Source: CAD feature listing. Evaluate the final solid. Frame: model axes, mm. Round coordinates to 2 decimals unless told otherwise and drop trailing zeros. Order: outer loops, then holes, each group sorted by start corner. A loop starts at its lowest first (then second) coordinate and runs counter-clockwise, first axis right, second up. Notation, with made-up numbers: (-6, 23.25) -> (18, 23.25) arc R21 cw to (18, 56.25) -> close; hole circle Ø3 at (-23.5, 47.5). An arc over 180 degrees is marked (long way). Answer as CSV lines item,"result". Start each with the question number.
(1) Section query C-C (z = -38.5). Count the separate pieces of the cut face and the enclosed holes in it, plus the area to 3 significant figures.
(2) Line query: line 1 along Y through (x, z) = (0, -21.25); line 2 along X through (y, z) = (100, -43); line 3 along X through (y, z) = (20, -22). Output: solid intervals per line, ascending. Write a range as from..to.
(3) Section query B-B (x = 80). Output: boundary loops of the cut face in (y, z).
(4) Section query A-A (y = 59). Output: boundary loops of the cut face in (x, z).
(5) Contact query for flat-ended pins moving along their axis: P1, Ø7.5, axis at x = -80, y = 100, coming from the +Z side; P2, Ø15, axis at x = -80, y = 100, coming from the +Z side; P3, Ø16.5, axis at x = 160, y = 100, coming from the +Z side. Output: stop coordinate, or through.
```python
from build123d import *

# Parameters (mm, degrees)
F0_W     = 400
F0_H     = 120
F0_R     = 12.7
F0_R_2   = 6.35
F1_DEPTH = 60
F3_D     = 12
F3_DEPTH = 80
F3_TIP   = 3.6051637142
F4_D     = 25.4
F4_DEPTH = 30
F4_TIP   = 7.6309298617
F5_D     = 12.7


with BuildPart() as f1:
    # F0 (on Top) → F1 (new body)
    with BuildSketch(Plane.XY):
        with Locations((0, 60)):
            Rectangle(F0_W, F0_H)
        with Locations((-80, 20)):
            Circle(F0_R, mode=Mode.SUBTRACT)
        with Locations((0, 20)):
            Circle(F0_R, mode=Mode.SUBTRACT)
        with Locations((80, 20)):
            Circle(F0_R, mode=Mode.SUBTRACT)
        with Locations((160, 20)):
            Circle(F0_R, mode=Mode.SUBTRACT)
        with Locations((-160, 100)):
            Circle(F0_R, mode=Mode.SUBTRACT)
        with Locations((-80, 100)):
            Circle(F0_R, mode=Mode.SUBTRACT)
        with Locations((0, 100)):
            Circle(F0_R, mode=Mode.SUBTRACT)
        with Locations((80, 100)):
            Circle(F0_R, mode=Mode.SUBTRACT)
        with Locations((160, 100)):
            Circle(F0_R, mode=Mode.SUBTRACT)
        with Locations((-160, 100)):
            Circle(F0_R)
        with Locations((-160, 100)):
            Circle(F0_R_2, mode=Mode.SUBTRACT)
        with Locations((-80, 100)):
            Circle(F0_R)
        with Locations((-80, 100)):
            Circle(F0_R_2, mode=Mode.SUBTRACT)
        with Locations((0, 100)):
            Circle(F0_R)
        with Locations((0, 100)):
            Circle(F0_R_2, mode=Mode.SUBTRACT)
        with Locations((80, 100)):
            Circle(F0_R)
        with Locations((80, 100)):
            Circle(F0_R_2, mode=Mode.SUBTRACT)
        with Locations((160, 100)):
            Circle(F0_R)
        with Locations((160, 100)):
            Circle(F0_R_2, mode=Mode.SUBTRACT)
        with Locations((80, 20)):
            Circle(F0_R)
        with Locations((80, 20)):
            Circle(F0_R_2, mode=Mode.SUBTRACT)
        with Locations((160, 20)):
            Circle(F0_R)
        with Locations((160, 20)):
            Circle(F0_R_2, mode=Mode.SUBTRACT)
        with Locations((0, 20)):
            Circle(F0_R)
        with Locations((0, 20)):
            Circle(F0_R_2, mode=Mode.SUBTRACT)
        with Locations((-80, 20)):
            Circle(F0_R)
        with Locations((-80, 20)):
            Circle(F0_R_2, mode=Mode.SUBTRACT)
        with Locations((-160, 100)):
            Circle(F0_R_2)
        with Locations((-80, 100)):
            Circle(F0_R_2)
        with Locations((0, 100)):
            Circle(F0_R_2)
        with Locations((80, 100)):
            Circle(F0_R_2)
        with Locations((160, 100)):
            Circle(F0_R_2)
        with Locations((80, 20)):
            Circle(F0_R_2)
        with Locations((160, 20)):
            Circle(F0_R_2)
        with Locations((0, 20)):
            Circle(F0_R_2)
        with Locations((-80, 20)):
            Circle(F0_R_2)
    extrude(amount=-F1_DEPTH)

    # F3
    with Locations(Plane.XZ):
        with Locations((-120, -12), (-120, -48), (120, -48), (120, -12)):
            Hole(F3_D / 2, depth=F3_DEPTH)
            with Locations((0, 0, -(F3_DEPTH + F3_TIP / 2))):  # 118° drill point
                Cone(0, F3_D / 2, F3_TIP, mode=Mode.SUBTRACT)

    # F4
    with Locations(Plane.XY):
        with Locations((-160, 100), (-80, 100), (0, 100), (80, 100), (160, 100), (160, 20), (80, 20), (0, 20), (-80, 20)):
            Hole(F4_D / 2, depth=F4_DEPTH)
            with Locations((0, 0, -(F4_DEPTH + F4_TIP / 2))):  # 118° drill point
                Cone(0, F4_D / 2, F4_TIP, mode=Mode.SUBTRACT)

    # F5 (through all)
    with Locations(Plane.XY):
        with Locations((-80, 20), (-80, 100), (-160, 100), (0, 100), (0, 20), (80, 20), (80, 100), (160, 100), (160, 20)):
            Hole(F5_D / 2)


solid = f1.part
```
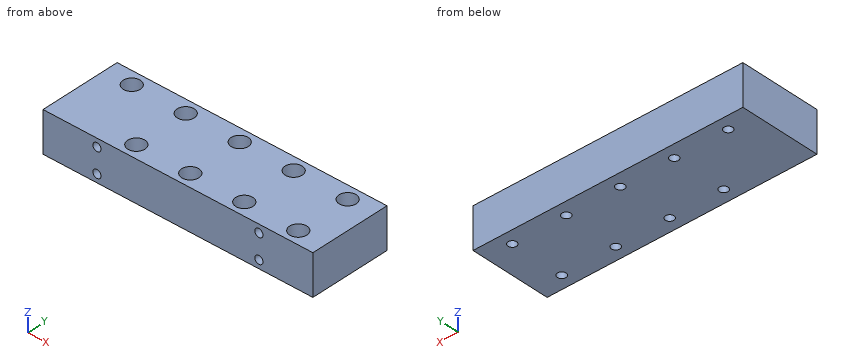
Answer block:
1,separate pieces,"1"
1,enclosed holes,"9"
1,area,"46,900 mm2"
2,line 1,"0..7.3, 32.7..87.3, 112.7..120"
2,line 2,"-200..-166.35, -153.65..-86.35, -73.65..-6.35, 6.35..73.65, 86.35..153.65, 166.35..200"
2,line 3,"-200..-92.7, -67.3..-12.7, 12.7..67.3, 92.7..147.3, 172.7..200"
3,outline,"(0, -60) -> (13.65, -60) -> (13.65, -33.82) -> (7.3, -30) -> (7.3, 0) -> (0, 0) -> close; (26.35, -60) -> (93.65, -60) -> (93.65, -33.82) -> (87.3, -30) -> (87.3, 0) -> (32.7, 0) -> (32.7, -30) -> (26.35, -33.82) -> close; (106.35, -60) -> (120, -60) -> (120, 0) -> (112.7, 0) -> (112.7, -30) -> (106.35, -33.82) -> close"
4,outline,"(-200, -60) -> (200, -60) -> (200, 0) -> (-200, 0) -> close; hole circle Ø12 at (-120, -48); hole circle Ø12 at (-120, -12); hole circle Ø12 at (120, -48); hole circle Ø12 at (120, -12)"
5,P1,"through"
5,P2,"z = -33.12"
5,P3,"z = -32.67"
